```python
from build123d import *

# Parameters (mm, degrees)
F0_R      = 4.75
F1_DEPTH  = 90
F2_R      = 2.7
F3_DEPTH  = 100
F4_R      = 3.175
F5_DEPTH  = 20
F6_R      = 3.15
F6_R_2    = 2.7
F7_DEPTH  = 10
F9_DEPTH  = 25
F11_DEPTH = 25
F14_DEPTH = 1.1
F15_SIZE  = 0.5


with BuildPart() as f1:
    # F0 (on Right) → F1 (new body)
    with BuildSketch(Plane.YZ):
        Circle(F0_R)
    extrude(amount=F1_DEPTH)

    # F2 (on Right) → F3 (cut)
    with BuildSketch(Plane.YZ):
        Circle(F2_R)
    extrude(amount=F3_DEPTH, mode=Mode.SUBTRACT)

    # F4 (on Right) → F5 (cut)
    with BuildSketch(Plane.YZ):
        Circle(F4_R)
    extrude(amount=F5_DEPTH, mode=Mode.SUBTRACT)

    # F6 (on face) → F7 (cut)
    with BuildSketch(Plane.YZ.offset(90)):
        Circle(F6_R)
        Circle(F6_R_2, mode=Mode.SUBTRACT)
    extrude(amount=-F7_DEPTH, mode=Mode.SUBTRACT)

    # F8 (on Front) → F9 (cut)
    with BuildSketch(Plane.XZ):
        with BuildLine():
            ThreePointArc((72.25, -1.1), (73.35, 0), (72.25, 1.1))
            Line((72.25, 1.1), (62.25, 1.1))
            ThreePointArc((62.25, 1.1), (61.15, 0), (62.25, -1.1))
            Line((62.25, -1.1), (72.25, -1.1))
        make_face()
    extrude(amount=-F9_DEPTH, mode=Mode.SUBTRACT)

    # F10 (on Top) → F11 (cut)
    with BuildSketch(Plane.XY):
        with BuildLine():
            ThreePointArc((62.25, 1.1), (61.15, 0), (62.25, -1.1))
            Line((62.25, -1.1), (63.75, -1.1))
            ThreePointArc((63.75, -1.1), (64.85, 0), (63.75, 1.1))
            Line((63.75, 1.1), (62.25, 1.1))
        make_face()
    extrude(amount=-F11_DEPTH, mode=Mode.SUBTRACT)

    # F13 (on offset) → F14 (cut, symmetric)
    with BuildSketch(Plane.YZ.offset(62.25)):
        with BuildLine():
            Line((0, 0), (0, -11.794144941))
            ThreePointArc((0, -11.794144941), (8.3397198661, -8.3397198661), (11.794144941, 0))
            Line((11.794144941, 0), (0, 0))
        make_face()
    extrude(amount=F14_DEPTH, both=True, mode=Mode.SUBTRACT)

    # F15
    f15_edges = [f1.edges().sort_by_distance(p)[0] for p in [
        (0, -4.75, 0),
    ]]
    chamfer(f15_edges, length=F15_SIZE)


solid = f1.part
```
Source: CAD feature listing. Evaluate the final solid. Frame: model axes, mm. A direction names the side the tool comes from. Give positions to 0.01 mm unless a question says otherwise; leave off trailing zeros. Order: outer loops, then holes, each group sorted by start corner. A loop starts at its lowest first (then second) coordinate and runs counter-clockwise, first axis right, second up.
(1) Material intervals for line 1 along Z through (x, y) = (83.25, 0); line 2 along Z through (x, y) = (9.5, 0) (3 decimals); line 3 along Y through (x, z) = (34, 0.25), sorted ascending.
(2) Section query B-B (x = 47). Return the cut outline in (y, z), plus the area to 3 significant figures.
(3) Contact query for flat-ended pins moving along their axis: P1, Ø1.7, axis at x = 67, y = 3, coming from the +Z side; P2, Ø3, axis at x = 72.5, z = -3, coming from the -Y side; P3, Ø3, axis at y = -1, z = -1, coming from the +X side; P4, Ø5, axis at y = 0, z = 0, coming from the -X side. Output: stop coordinate, or through.
(4) Pull-direction query (X, two-part tool) for faces 1 (the face through (68, 4, -1.1)), 2 (the face through (0, -2, -3)), 3 (the face through (49.58, -1.99, 1.825)); classes: +X half, -X half, draft (parallel to the pull), parting line (faces both ways), or undercut.
(5) Access query for faces 4 (the face through (63.35, 2.4, -2.4)), 5 (the face through (67, 4, 1.1)), 6 (the face through (64.85, -0.02, -3.59)). Directions: +Z, -Z, +X, -X, +Y, -Y. A direction counts if a zero-diameter tool reaches every point of the face in a straight line with its end or side. Return the directions, or none.
(6) Section query A-A (x = 81). Return the cut outline in (y, z), plus the area to 3 significant figures.
Outcome:
1. line 1: z = -4.75 to -3.15, 3.15 to 4.75
1. line 2: z = -4.75 to -3.175, 3.175 to 4.75
1. line 3: y = -4.74 to -2.69, 2.69 to 4.74
2. outline: circle Ø9.5 at (0, 0); hole circle Ø5.4 at (0, 0)
2. area: 48.0 mm2
3. P1: stops at z = 4.24
3. P2: stops at y = -4.51
3. P3: stops at x = 80
3. P4: passes through
4. face 1: undercut
4. face 2: -X half
4. face 3: draft
5. face 4: -Z, +Y
5. face 5: +Y
5. face 6: -Z
6. outline: circle Ø9.5 at (0, 0); hole circle Ø6.3 at (0, 0)
6. area: 39.7 mm2
